Input: dimensioned drawing with shaded views. Units: mm. Origin: part minimum x, y, z. A direction names the side the tool comes from. Round coordinates to 2 decimals unless told otherwise and drop trailing zeros. Loops run counter-clockwise (first coordinate to the right, second up) from the corner with the lowest first, then second, coordinate; pieces in that order, holes last. Notation, with made-up numbers: M -20.75,85.5 L 0.25,85.5 A25 cw 0.25,104.5 Z; hole C -13.75,2.25 d11. An arc over 180 degrees is marked long. Answer as a JSON object with one key per item and string values.
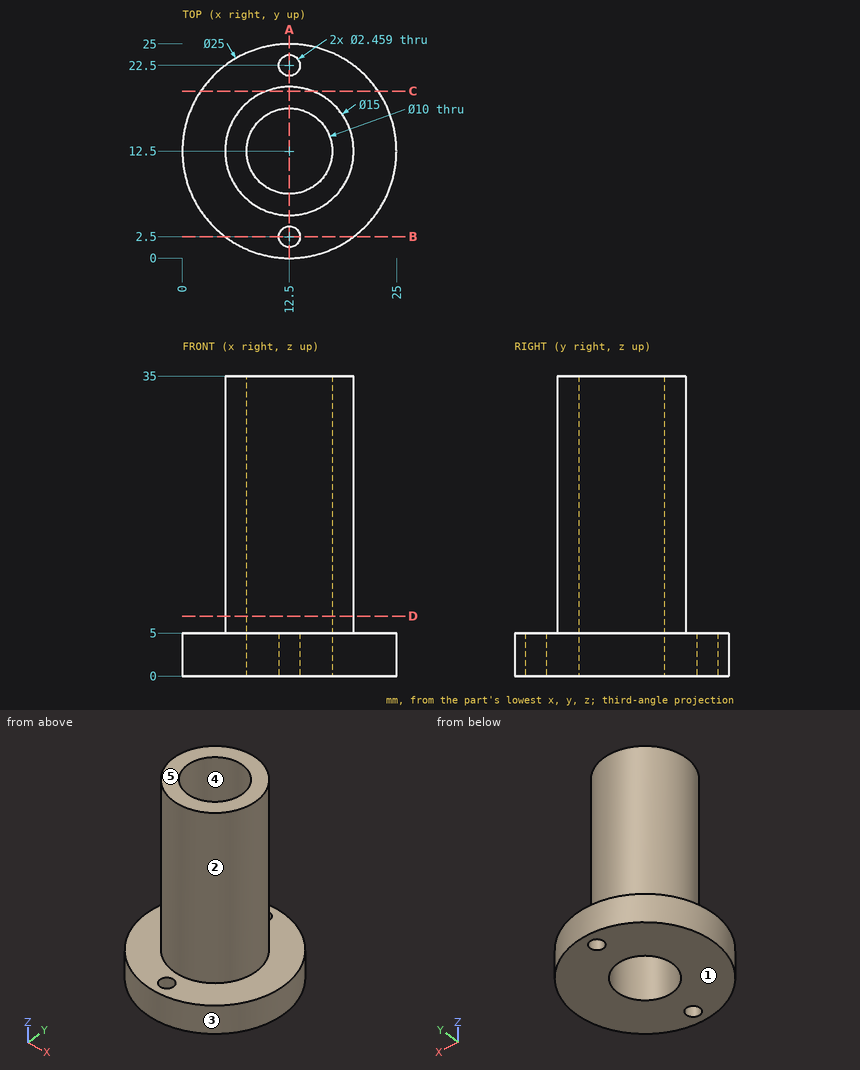
Item 1: Section C-C on y = 19.5. Return the cut outline in (x, z).
Answer sheet:
{"outline": "M 2.14,0 L 22.86,0 L 22.86,5 L 15.19,5 L 15.19,35 L 9.81,35 L 9.81,5 L 2.14,5 Z"}
Item 2: Pull-direction query (X, two-part tool) for the marked faces 3, 4 and 5; classes: pulls with the +X half, pulls with the -X half, needs draft (parallel to the pull), parting line crosses it, or undercut.
Answer sheet:
{"face 3": "parting line crosses it", "face 4": "undercut", "face 5": "needs draft"}
Item 3: Access query for the marked faces 1 and 2. Directions: +Z, -Z, +X, -X, +Y, -Y. A direction counts if a zero-diameter tool reaches every point of the face in a straight line with its end or side. Return the directions, or none.
Answer sheet:
{"face 1": "-Z, +X, -X, +Y, -Y", "face 2": "+Z"}
Item 4: Section B-B on y = 2.5. Return the cut outline in (x, z).
Answer sheet:
{"outline": "M 5,0 L 11.27,0 L 11.27,5 L 5,5 Z; M 13.73,0 L 20,0 L 20,5 L 13.73,5 Z"}
Item 5: Contact query for flat-ended pins moving along their axis: pin 1 Ø10 at (x, z) = (20, 5.5) entering from +Y; pin 2 Ø3 at (x, z) = (17, 10.5) entering from -Y; pin 3 Ø4 at (y, z) = (18.5, 29) entering from -X; pin 4 Ø2 at (x, y) = (12.5, 2.5) entering from +Z. Output: stop coordinate, or through.
Answer sheet:
{"pin 1": "stops at y = 24.74", "pin 2": "stops at y = 5.63", "pin 3": "stops at x = 6.16", "pin 4": "passes through"}
Item 6: Line query: probe 1 along Y at (x, z) = (12.5, 23); probe 2 along Y at (x, z) = (12.5, 2.8); probe 3 along Z at (x, y) = (15.75, 19.75). Output: solid intervals per line, ascending. Write a range as from..to.
Answer sheet:
{"probe 1": "y = 5..7.5, 17.5..20", "probe 2": "y = 0..1.27, 3.73..7.5, 17.5..21.27, 23.73..25", "probe 3": "z = 0..5"}
Item 7: Section D-D on z = 7. Return the cut outline in (x, y).
Answer sheet:
{"outline": "C 12.5,12.5 d15; hole C 12.5,12.5 d10"}
Item 8: Section A-A on x = 12.5. Return the cut outline in (y, z).
Answer sheet:
{"outline": "M 0,0 L 1.27,0 L 1.27,5 L 0,5 Z; M 3.73,0 L 7.5,0 L 7.5,35 L 5,35 L 5,5 L 3.73,5 Z; M 17.5,0 L 21.27,0 L 21.27,5 L 20,5 L 20,35 L 17.5,35 Z; M 23.73,0 L 25,0 L 25,5 L 23.73,5 Z"}
